Can you work these out from the model? Positions are in its coordinate system, mm. Coordinates: 2 decimals unless noted, no trailing zeros. Write each loop counter-clockwise with the first axis right and the second up, starting at its lowest first coordinate (ties: lowest second). Pieces come first, ordered by that corner, then holes. Notation, with made-up numbers: (63, 48) - (77, 48) arc R20 ccw to (77, 74) - close; hole circle Ø6 at (37.5, 16). An arc over 180 degrees is marked (long way). Write each question's results on one line, items separated by ' | '. Start each with the question number.
```python
from build123d import *

# Parameters (mm, degrees)
ESQUISSE1_R        = 4
ESQUISSE1_R_2      = 1.5
BOSS_EXTRU_1_DEPTH = 5
CONG_1_R           = 10
CONG_2_R           = 20


with BuildPart() as part:
    # Esquisse1 → Boss.-Extru.1 (new body)
    with BuildSketch(Plane.XY):
        Polygon((-21.5, 0), (-25, 0), (-25, -5), (-30, -5), (-30, 0), (-35, 0), (-35, 20), (-45, 60), (-45, 95.993420768), (-35, 95.993420768), (-10, 95.993420768), (8.893717408, 95.993420768), (70.442895342, 202.763784424), (70.442895342, 250), (97.672831982, 250), (130, 250), (130, 255), (135, 255), (135, 250), (138.5, 250), (138.5, 247), (137.4, 247), (137.4, 244.7), (138.5, 244.7), (138.5, 240), (141.5, 240), (141.5, 244.7), (142.6, 244.7), (142.6, 247), (141.5, 247), (141.5, 250), (145, 250), (145, 255), (150, 255), (150, 250), (190, 250), (190, 210), (132.327168018, 210), (35, 41.164972924), (35, 0), (30, 0), (30, -5), (25, -5), (25, 0), (21.5, 0), (21.5, 3), (22.6, 3), (22.6, 5.3), (21.5, 5.3), (21.5, 10), (18.5, 10), (18.5, 5.3), (17.4, 5.3), (17.4, 3), (18.5, 3), (18.5, 0), (15, 0), (15, -5), (10, -5), (10, 0), (-10, 0), (-10, -5), (-15, -5), (-15, 0), (-18.5, 0), (-18.5, 3), (-17.4, 3), (-17.4, 5.3), (-18.5, 5.3), (-18.5, 10), (-21.5, 10), (-21.5, 5.3), (-22.6, 5.3), (-22.6, 3), (-21.5, 3), align=None)
        with Locations((115, 230)):
            Circle(ESQUISSE1_R, mode=Mode.SUBTRACT)
        with Locations((175, 230)):
            Circle(ESQUISSE1_R, mode=Mode.SUBTRACT)
        with Locations((85, 230)):
            Circle(ESQUISSE1_R, mode=Mode.SUBTRACT)
        with Locations((-24.543125869, 83.023041686)):
            Circle(ESQUISSE1_R_2, mode=Mode.SUBTRACT)
        Polygon((-29.672175025, 80.799788495), (-32.886113073, 76.969566279), (-29.055890858, 73.755628231), (-25.841952809, 77.585850447), align=None, mode=Mode.SUBTRACT)
        Polygon((-23.244298928, 88.460232926), (-20.03036088, 92.290455142), (-16.200138664, 89.076517093), (-19.414076712, 85.246294878), align=None, mode=Mode.SUBTRACT)
    extrude(amount=BOSS_EXTRU_1_DEPTH)

    # Congé1
    cong_1_edges = [part.edges().sort_by_distance(p)[0] for p in [
        (-35, 20, 2.5),
        (-45, 60, 2.5),
        (-45, 95.993420768, 2.5),
    ]]
    fillet(cong_1_edges, radius=CONG_1_R)

    # Congé2
    cong_2_edges = [part.edges().sort_by_distance(p)[0] for p in [
        (35, 41.164972924, 2.5),
        (132.327168018, 210, 2.5),
        (190, 210, 2.5),
        (70.442895342, 250, 2.5),
        (190, 250, 2.5),
        (8.893717408, 95.993420768, 2.5),
        (70.442895342, 202.763784424, 2.5),
    ]]
    fillet(cong_2_edges, radius=CONG_2_R - 0.0001)  # a hair under: the kernel refuses the full size


solid = part.part
```
Q1. I'm going to push flat-ended pins straight in: pin 1 Ø1.5 at (y, z) = (10, 2.5) entering from -X; pin 2 Ø2 at (y, z) = (170.5, 4) entering from +X; pin 3 Ø2.5 at (y, z) = (2, 2.5) entering from +X. Where does each tip first touch, or does it pass through?
Q2. If we section it at D-D (y = 114.5): Please give me the cut outline in (x, z), then the cut area to 3 significant figures.
Q3. I need wall thicknesses on line 1 along Y through (x, z) = (85, 1.85); line 2 along Y through (x, z) = (111.5, 4.05); line 3 along X through (y, z) = (55.5, 4.2) (3 decimals). Which ranges of each line are inside material? Lowest first, please. Write a range as from..to.
Q4. Thinking about a two-plate mould opening in X: for faces 1 (the face through (117.15, 233.373, 2.465)), 2 (the face through (178.815, 231.201, 2.465)), 3 (the face through (56, 135, 5)), 4 (the face through (7.216, 98.603, 2.535)), which applies, pulls with the +X half, pulls with the -X half, needs draft (parallel to the pull), parting line crosses it, or undercut?
Q5. If we section it at B-B (x = 175): Please give me the cut outline in (y, z).
Q6. If we section it at A-A (x = 85): Please give me the cut outline in (y, z).
Q7. If we section it at C-C (z = 2.45): Count the separate pieces of the cut face and the enclosed holes in it, then the cut area to 3 significant figures.
Answer list:
1) pin 1: stops at x = -35 | pin 2: stops at x = 110.13 | pin 3: stops at x = 35
2) outline: (19.56, 0) - (77.27, 0) - (77.27, 5) - (19.56, 5) - close | area: 289 mm2
3) line 1: y = 127.9..226, 234..249.25 | line 2: y = 173.87..228.06, 231.94..250 | line 3: x = -43.875..43.264
4) face 1: undercut | face 2: undercut | face 3: needs draft | face 4: pulls with the -X half
5) outline: (210.64, 0) - (226, 0) - (226, 5) - (210.64, 5) - close; (234, 0) - (249.36, 0) - (249.36, 5) - (234, 5) - close
6) outline: (127.9, 0) - (226, 0) - (226, 5) - (127.9, 5) - close; (234, 0) - (249.25, 0) - (249.25, 5) - (234, 5) - close
7) separate pieces: 1 | enclosed holes: 6 | area: 19,100 mm2
